```python
from build123d import *

# Parameters (mm, degrees)
F1_DEPTH    = 3.4544
F2_R        = 2.59715
F2_R_2      = 1.98755
F3_DEPTH    = 3.4554
F4_C1_SIZE2 = 0.127
F4_C1_SIZE  = 0.2199704526
F4_C2_SIZE2 = 0.127
F4_C2_SIZE  = 0.2199704526
F4_C3_SIZE2 = 0.127
F4_C3_SIZE  = 0.2199704526
F4_C4_SIZE2 = 0.127
F4_C4_SIZE  = 0.2199704526
F5_R        = 0.381


with BuildPart() as f1:
    # F0 (on Front) → F1 (new body)
    with BuildSketch(Plane.XZ):
        with BuildLine():
            Line((3.9421045586, -3.9184314079), (4.6496617871, 3.0454783394))
            ThreePointArc((4.6496617871, 3.0454783394), (0, 8.1915), (-4.6496617871, 3.0454783394))
            Line((-4.6496617871, 3.0454783394), (-3.9421045586, -3.9184314079))
            ThreePointArc((-3.9421045586, -3.9184314079), (0, -7.4803), (3.9421045586, -3.9184314079))
        make_face()
    extrude(amount=-F1_DEPTH)

    # F2 (on face) → F3 (cut, through all)
    with BuildSketch(Plane.XZ):
        with Locations((0, 3.5179)):
            Circle(F2_R)
        with Locations((0, -3.5433)):
            Circle(F2_R_2)
    extrude(amount=-F3_DEPTH, mode=Mode.SUBTRACT)

    # F4: chamfer of 0.127 x 0.2199704526 on 4 edges, made by hand

    # F4_c1
    f4_c1_edges = [f1.edges().sort_by_distance(p)[0] for p in [
        (-1.98755, 0, -3.5433),
    ]]
    f4_c1_side = f1.faces().sort_by_distance((-1.99009, 0, -3.5433))[0]
    chamfer(f4_c1_edges, length=F4_C1_SIZE, length2=F4_C1_SIZE2, reference=f4_c1_side)

    # F4_c2
    f4_c2_edges = [f1.edges().sort_by_distance(p)[0] for p in [
        (-2.59715, 0, 3.5179),
    ]]
    f4_c2_side = f1.faces().sort_by_distance((-2.59969, 0, 3.5179))[0]
    chamfer(f4_c2_edges, length=F4_C2_SIZE, length2=F4_C2_SIZE2, reference=f4_c2_side)

    # F4_c3
    f4_c3_edges = [f1.edges().sort_by_distance(p)[0] for p in [
        (-1.98755, 3.4544, -3.5433),
    ]]
    f4_c3_side = f1.faces().sort_by_distance((-1.98755, 3.45186, -3.5433))[0]
    chamfer(f4_c3_edges, length=F4_C3_SIZE, length2=F4_C3_SIZE2, reference=f4_c3_side)

    # F4_c4
    f4_c4_edges = [f1.edges().sort_by_distance(p)[0] for p in [
        (-2.59715, 3.4544, 3.5179),
    ]]
    f4_c4_side = f1.faces().sort_by_distance((-2.59969, 3.4544, 3.5179))[0]
    chamfer(f4_c4_edges, length=F4_C4_SIZE, length2=F4_C4_SIZE2, reference=f4_c4_side)

    # F5
    f5_edges = [f1.edges().sort_by_distance(p)[0] for p in [
        (0, 0, -7.4803),
        (0, 3.4544, -7.4803),
        (4.295883, 3.4544, -0.436477),
        (0, 3.4544, 8.1915),
        (-4.295883, 3.4544, -0.436477),
        (4.295883, 0, -0.436477),
        (0, 0, 8.1915),
        (-4.295883, 0, -0.436477),
    ]]
    fillet(f5_edges, radius=F5_R)


solid = f1.part
```
Source: CAD feature listing. Evaluate the final solid. Frame: model axes, mm. Coordinates: 2 decimals unless noted, no trailing zeros. Loops run counter-clockwise (first coordinate to the right, second up) from the corner with the lowest first, then second, coordinate; pieces in that order, holes last. Notation, with made-up numbers: (53.25, 23) -> (81.25, 23) arc R23 ccw to (81.25, 59) -> close; hole circle Ø9 at (78.5, 88.5). An arc over 180 degrees is marked (long way). One line per item, written item: value. Start each with the question number.
Q1. Line query: line 1 along Z through (x, y) = (0, 0.85); line 2 along Z through (x, y) = (-1.5, 1.15); line 3 along X through (y, z) = (1.15, 1.25). Output: solid intervals per line, ascending.
Q2. Section query C-C, the plane x = -1. Give the number of separate pieces and of enclosed holes in the cut face, and give its area (3 significant figures).
Q3. Section query A-A, the plane x = 0. Return the cut outline in (y, z), and give its area (3 significant figures).
Q4. Section query B-B, the plane y = 0.85. Return the cut outline in (x, z).
Q5. Contact query for flat-ended pins moving along their axis: P1, Ø1.5, axis at y = 2, z = -2, coming from the -X side; P2, Ø4.5, axis at x = 0, z = -3.54, coming from the -Y side. Output: stop coordinate, or through.
Q6. Mould query, pull axis Z, two halves, no side actions, for faces 1 (the face through (0, 3.454, 0)), 2 (the face through (-4.18, 0.11, -0.47)), 3 (the face through (-0.431, 1.659, -5.484)). Classes: pulls with the +Z half, pulls with the -Z half, needs draft (parallel to the pull), parting line crosses it, or undercut.
Results:
1. line 1: -7.48 to -5.53, -1.56 to 0.92, 6.12 to 8.19
1. line 2: -7.19 to -4.85, -2.24 to 1.4, 5.64 to 7.94
1. line 3: -4.47 to -1.27, 1.27 to 4.47
2. separate pieces: 3
2. enclosed holes: 0
2. area: 24.6 mm^2
3. outline: (0, -7.1) arc R0.38 ccw to (0.38, -7.48) -> (3.07, -7.48) arc R0.38 ccw to (3.45, -7.1) -> (3.45, -5.66) -> (3.23, -5.53) -> (0.13, -5.53) -> (0, -5.75) -> close; (0, -1.34) -> (0.13, -1.56) -> (3.23, -1.56) -> (3.45, -1.43) -> (3.45, 0.7) -> (3.33, 0.92) -> (0.13, 0.92) -> (0, 0.7) -> close; (0, 6.34) -> (0.13, 6.12) -> (3.33, 6.12) -> (3.45, 6.34) -> (3.45, 7.81) arc R0.38 ccw to (3.07, 8.19) -> (0.38, 8.19) arc R0.38 ccw to (0, 7.81) -> close
3. area: 22.2 mm^2
4. outline: (-4.65, 3.05) -> (-3.94, -3.92) arc R3.96 ccw to (3.94, -3.92) -> (4.65, 3.05) arc R4.67 ccw (long way) to start; hole circle Ø5.19 at (0, 3.52); hole circle Ø3.98 at (0, -3.54)
5. P1: x = -4.21
5. P2: y = 0
6. face 1: needs draft
6. face 2: pulls with the -Z half
6. face 3: undercut
